The listing builds one solid part. Answer for the finished solid, in the listing's coordinates (mm). Face numbers are marked on the shaded views. A direction names the side the tool comes from. Coordinates: 2 decimals unless noted, no trailing zeros. Order: outer loops, then holes, each group sorted by start corner. A loop starts at its lowest first (then second) coordinate and runs counter-clockwise, first axis right, second up. Notation, with made-up numbers: (32.5, 47.25) - (54.5, 47.25) arc R8 ccw to (54.5, 58.25) - close; hole circle Ø8 at (48.25, 41.5). An arc over 180 degrees is marked (long way). Use one line per item in the form item = value. Start each with the question number.
Item 1: Section B-B, the plane y = -32.5 is taken. Write down the section's boundary in (x, z), and give its area (3 significant figures).
Item 2: The mould has two halves that part along Z. Classify the marked faces 3, 4, 5 and 6: released by +Z, released by -Z, zero draft, split by the parting line, or undercut.
Item 3: Section A-A, the plane x = 215.9 is taken. Write down the section's boundary in (y, z), and give its area (3 significant figures).
Item 4: Each of these flat-tipped pins is pushed along its axis until it touches: pin 1 Ø5 at (x, z) = (168.5, -117.5) entering from +Y; pin 2 Ø8 at (x, y) = (86.5, -119) entering from +Z. Where does it stop, or does it pass through?
Item 5: Section D-D, the plane y = -91 is taken. Write down the section's boundary in (x, z).
Item 6: Section C-C, the plane z = -88.9 is taken. Write down the section's boundary in (x, y).
Item 7: A tool of negligible diameter and unlimited length cuts with its end or side. For the marked faces 1 and 2, from which of +Z, -Z, +X, -X, +Y, -Y can it reach the whole face along a straight path? Write none if from no direction.
Item 8: Consider line 1 along X through (y, z) = (-138.5, -88.9); line 2 along X through (y, z) = (-83, -88.9); line 3 along Z through (x, y) = (53, -36.5). Determine where each line is inside the solid, lowest interval first. Write a range as [from, to].
from build123d import *

# Parameters (mm, degrees)
SKETCH1_W           = 304.8
SKETCH1_H           = 177.8
SKETCH1_W_2         = 254
SKETCH1_H_2         = 127
BOSS_EXTRUDE2_DEPTH = 152.4
SKETCH4_W           = 127
SKETCH4_H           = 127
SKETCH4_R           = 25.4
BOSS_EXTRUDE3_DEPTH = 152.4
SKETCH5_W           = 127
SKETCH5_H           = 127
CUT_EXTRUDE1_DEPTH  = 50.8
SKETCH10_W          = 127
SKETCH10_H          = 127
CUT_EXTRUDE2_DEPTH  = 114.3


with BuildPart() as part:
    # Sketch1 → Boss-Extrude2 (new body)
    with BuildSketch(Plane(origin=(0, 0, 0), x_dir=(1, 0, 0), z_dir=(0, 1, 0))):
        with Locations((152.4, 88.9)):
            Rectangle(SKETCH1_W, SKETCH1_H)
        with Locations((152.4, 88.9)):
            Rectangle(SKETCH1_W_2, SKETCH1_H_2, mode=Mode.SUBTRACT)
    extrude(amount=-BOSS_EXTRUDE2_DEPTH)

    # Sketch4 → Boss-Extrude3 (add)
    # profile 1 of 2: a face of its own
    with BuildSketch(Plane(origin=(0, 0, 0), x_dir=(1, 0, 0), z_dir=(0, 1, 0))):
        with Locations((215.9, 88.9)):
            Rectangle(SKETCH4_W, SKETCH4_H)
        with Locations(Location((215.9, 88.9, 0), (0, 0, 270))):
            Circle(SKETCH4_R, mode=Mode.SUBTRACT)
    # profile 2 of 2: a face of its own
    with BuildSketch(Plane(origin=(0, 0, 0), x_dir=(1, 0, 0), z_dir=(0, 1, 0))):
        with Locations((88.9, 88.9)):
            Rectangle(SKETCH4_W, SKETCH4_H)
        with Locations(Location((88.9, 88.9, 0), (0, 0, 270))):
            Circle(SKETCH4_R, mode=Mode.SUBTRACT)
    extrude(amount=-BOSS_EXTRUDE3_DEPTH)

    # Sketch5 → Cut-Extrude1 (cut)
    with BuildSketch(Plane(origin=(0, 0, 0), x_dir=(1, 0, 0), z_dir=(0, 1, 0))):
        with Locations((88.9, 88.9)):
            Rectangle(SKETCH5_W, SKETCH5_H)
    extrude(amount=-CUT_EXTRUDE1_DEPTH, mode=Mode.SUBTRACT)

    # Sketch10 → Cut-Extrude2 (cut)
    with BuildSketch(Plane(origin=(0, 0, 0), x_dir=(1, 0, 0), z_dir=(0, 1, 0))):
        with Locations((215.9, 88.9)):
            Rectangle(SKETCH10_W, SKETCH10_H)
    extrude(amount=-CUT_EXTRUDE2_DEPTH, mode=Mode.SUBTRACT)


solid = part.part
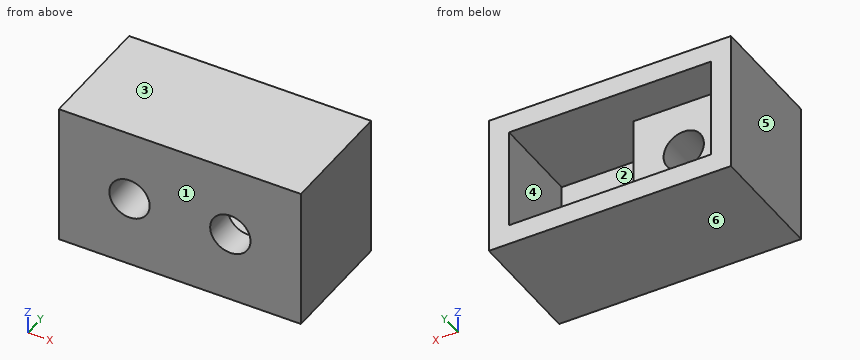
Response:
q1.outline = (0, -177.8) - (304.8, -177.8) - (304.8, 0) - (0, 0) - close; hole (25.4, -152.4) - (279.4, -152.4) - (279.4, -25.4) - (25.4, -25.4) - close
q1.area = 21,900 mm2
q2.face_3 = released by +Z
q2.face_4 = undercut
q2.face_5 = zero draft
q2.face_6 = released by -Z
q3.outline = (-152.4, -177.8) - (0, -177.8) - (0, -152.4) - (-114.3, -152.4) - (-114.3, -114.3) - (-152.4, -114.3) - close; (-152.4, -63.5) - (-114.3, -63.5) - (-114.3, -25.4) - (0, -25.4) - (0, 0) - (-152.4, 0) - close
q3.area = 10,600 mm2
q4.pin_1 = -114.3
q4.pin_2 = 0
q5.outline = (0, -177.8) - (304.8, -177.8) - (304.8, 0) - (0, 0) - close; hole circle Ø50.8 at (88.9, -88.9); hole (152.4, -152.4) - (279.4, -152.4) - (279.4, -25.4) - (152.4, -25.4) - close
q6.outline = (0, -152.4) - (63.5, -152.4) - (63.5, -50.8) - (25.4, -50.8) - (25.4, 0) - (0, 0) - close; (114.3, -152.4) - (190.5, -152.4) - (190.5, -114.3) - (152.4, -114.3) - (152.4, -50.8) - (114.3, -50.8) - close; (241.3, -152.4) - (304.8, -152.4) - (304.8, 0) - (279.4, 0) - (279.4, -114.3) - (241.3, -114.3) - close
q7.face_1 = +Z, -Z, +X, -X, -Y
q7.face_2 = +Y
q8.line_1 = [0, 63.5], [114.3, 190.5], [241.3, 304.8]
q8.line_2 = [0, 63.5], [114.3, 152.4], [279.4, 304.8]
q8.line_3 = [-177.8, -152.4], [-25.4, 0]
